Source: CAD feature listing. Evaluate the final solid. Frame: model axes, mm. Face numbers are marked on the shaded views. Round coordinates to 2 decimals unless told otherwise and drop trailing zeros. Loops run counter-clockwise (first coordinate to the right, second up) from the corner with the lowest first, then second, coordinate; pieces in that order, holes last.
Item 1: Section query A-A on y = 16. Return loops of the section in (x, z).
Item 2: Section query C-C on x = 45. Return loops of the section in (y, z), then the cut area to 3 significant figures.
Item 3: Ray query, L1, parallel to X at y = 12.5, z = -19.5; L2, parallel to Y at x = 123, z = -81; L3, parallel to Z at x = 99, y = 11.5. Return the intervals inside material, ascending.
Item 4: Pull-direction query (X, two-part tool) for the marked faces 1 and 2; classes: released by +X, released by -X, zero draft, split by the parting line, or undercut.
Item 5: First-contact query: P1, Ø2, axis at x = 181, y = 16.5, coming from the +Z side; P2, Ø1.2, axis at x = 181, y = 13, coming from the -Z side; P3, Ø5, axis at y = 16, z = -100, coming from the +X side; P4, Ø12, axis at x = 71, z = -106.5, coming from the -Y side. Flat tips, straight axial feed; report the tip coordinate or a pass-through.
Item 6: Section query B-B on z = -26. Return loops of the section in (x, y), then the cut area to 3 significant figures.
Item 7: Section query D-D on z = -76.5. Return loops of the section in (x, y).
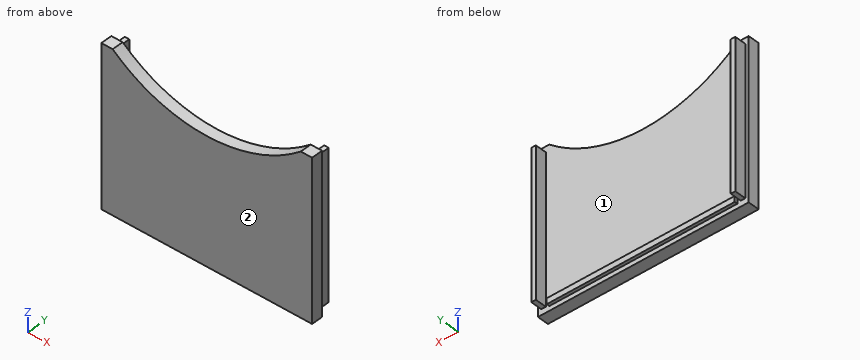
```python
from build123d import *

# Parameters (mm, degrees)
SKETCH1_W           = 186
SKETCH1_H           = 140
BOSS_EXTRUDE1_DEPTH = 10
CUT_EXTRUDE5_DEPTH  = 234.015020975
SKETCH4_W           = 166
SKETCH4_H           = 5
BOSS_EXTRUDE3_DEPTH = 2.6416
SKETCH6_W           = 4
SKETCH6_H           = 130
BOSS_EXTRUDE4_DEPTH = 10
SKETCH7_W           = 4
SKETCH7_H           = 130
BOSS_EXTRUDE5_DEPTH = 10


with BuildPart() as part:
    # Sketch1 → Boss-Extrude1 (new body)
    with BuildSketch(Plane(origin=(0, 0, 0), x_dir=(1, 0, 0), z_dir=(0, 1, 0))):
        with Locations((93, 70)):
            Rectangle(SKETCH1_W, SKETCH1_H)
    extrude(amount=BOSS_EXTRUDE1_DEPTH)

    # Sketch5 → Cut-Extrude5 (cut, through all)
    with BuildSketch(Plane(origin=(0, 10, 0), x_dir=(1, 0, 0), z_dir=(0, 1, 0))):
        with BuildLine():
            Line((176, 0), (10, 0))
            ThreePointArc((10, 0), (93, 30), (176, 0))
        make_face()
    extrude(amount=-CUT_EXTRUDE5_DEPTH, mode=Mode.SUBTRACT)

    # Sketch4 → Boss-Extrude3 (add)
    with BuildSketch(Plane(origin=(0, 10, 0), x_dir=(1, 0, 0), z_dir=(0, 1, 0))):
        with Locations((93, 133.5)):
            Rectangle(SKETCH4_W, SKETCH4_H)
    extrude(amount=BOSS_EXTRUDE3_DEPTH)

    # Sketch6 → Boss-Extrude4 (add)
    with BuildSketch(Plane(origin=(0, 10, 0), x_dir=(1, 0, 0), z_dir=(0, 1, 0))):
        with Locations((181, 70)):
            Rectangle(SKETCH6_W, SKETCH6_H)
    extrude(amount=BOSS_EXTRUDE4_DEPTH)

    # Sketch7 → Boss-Extrude5 (add)
    with BuildSketch(Plane(origin=(0, 10, 0), x_dir=(1, 0, 0), z_dir=(0, 1, 0))):
        with Locations((5, 70)):
            Rectangle(SKETCH7_W, SKETCH7_H)
    extrude(amount=BOSS_EXTRUDE5_DEPTH)


solid = part.part
```
Data:
1. outline: (3, -135) - (7, -135) - (7, -5) - (3, -5) - close; (179, -135) - (183, -135) - (183, -5) - (179, -5) - close
2. outline: (0, -140) - (10, -140) - (10, -136) - (12.64, -136) - (12.64, -131) - (10, -131) - (10, -20.8) - (0, -20.8) - close
2. area: 1,210 mm2
3. L1: x = 3 to 7, 179 to 183
3. L2: y = 0 to 10
3. L3: z = -136 to -131
4. face 1: undercut
4. face 2: zero draft
5. P1: stops at z = -5
5. P2: stops at z = -135
5. P3: stops at x = 183
5. P4: stops at y = 0
6. outline: (0, 0) - (61.02, 0) - (61.02, 10) - (7, 10) - (7, 20) - (3, 20) - (3, 10) - (0, 10) - close; (124.98, 0) - (186, 0) - (186, 10) - (183, 10) - (183, 20) - (179, 20) - (179, 10) - (124.98, 10) - close
6. area: 1,300 mm2
7. outline: (0, 0) - (186, 0) - (186, 10) - (183, 10) - (183, 20) - (179, 20) - (179, 10) - (7, 10) - (7, 20) - (3, 20) - (3, 10) - (0, 10) - close
